Print and shaded views of the part. All mm, measured from the part's lowest x, y and z. Coordinates: 2 decimals unless noted, no trailing zeros. Order: outer loops, then holes, each group sorted by start corner. A loop starts at its lowest first (then second) coordinate and runs counter-clockwise, first axis right, second up. Notation, with made-up numbers: (28.5, 51.5) -> (32.5, 51.5) arc R27 cw to (32.5, 81.5) -> close; hole circle Ø7 at (-30, 8). An arc over 180 degrees is marked (long way). Return JSON: item names as keys, results as strings. Group by question number.
1) Cut at B-B (y = 0.5). State how many separate pieces and enclosed holes the cut face has, and give its area (3 significant figures).
2) Cut at A-A (x = 145). Write the cut outline in (y, z), and give its area (3 significant figures).
3) Probe line 1 (X direction, y = 2.7, z = 4.75); line 2 (Z direction, x = 145, y = 1.3); line 3 (X direction, y = 2.85, z = 6.75). List the from-to ranges inside material, lowest first.
4) Flat gauge pins, fed straight in: pin 1 (1.5 mm diameter, centred on y = 2.5, z = 7.5, fed in from -X); pin 2 (5.5 mm diameter, centred on x = 194, z = 5, fed in from -Y). Where does each tip first touch, or does it go through?
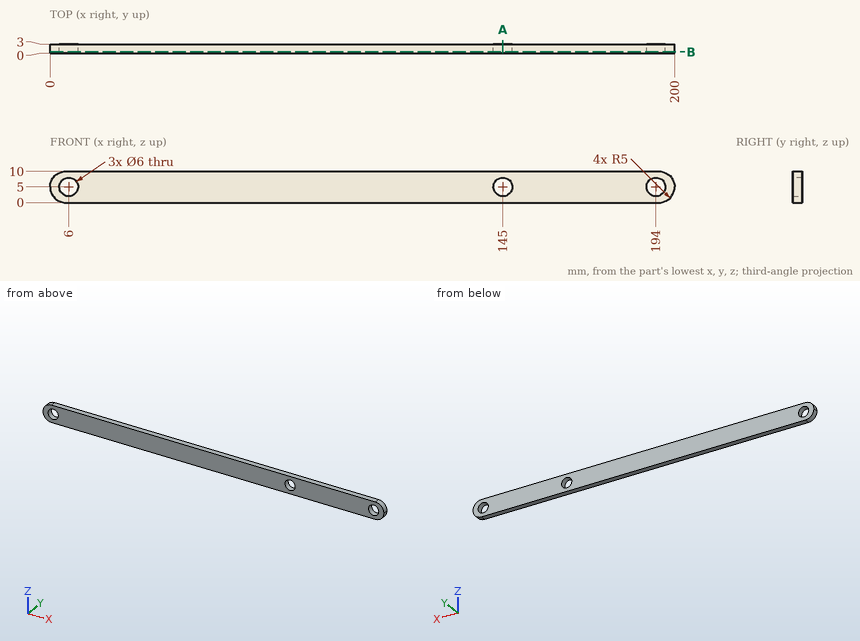
Answers below:
{
 "1": {"separate pieces": "1", "enclosed holes": "3", "area": "1,890 mm^2"},
 "2": {"outline": "(0, 0) -> (3, 0) -> (3, 2) -> (0, 2) -> close; (0, 8) -> (3, 8) -> (3, 10) -> (0, 10) -> close", "area": "12.0 mm^2"},
 "3": {"line 1": "x = 0.01 to 3.01, 8.99 to 142.01, 147.99 to 191.01, 196.99 to 199.99", "line 2": "z = 0 to 2, 8 to 10", "line 3": "x = 0.32 to 3.56, 8.44 to 142.56, 147.44 to 191.56, 196.44 to 199.68"},
 "4": {"pin 1": "stops at x = 0.32", "pin 2": "passes through"}
}
